Read the model definition and answer for the solid it produces. Units are mm, in the model's axes. Give positions to 0.01 mm unless a question says otherwise; leave off trailing zeros. Answer as a JSON object with one key per item and string values. Group by question number.
```python
from build123d import *

# Parameters (mm, degrees)
SKETCH2_R          = 5.55625
CUT_EXTRUDE1_DEPTH = 141.819693743
CIRPATTERN1_COUNT  = 4
CHAMFER1_SIZE      = 0.508
CHAMFER1_SIZE2     = 3.302
CHAMFER2_SIZE      = 1.5875
FILLET1_R          = 0.762


with BuildPart() as part:
    # Sketch1 → Revolve1 (revolve)
    with BuildSketch(Plane.XY, mode=Mode.PRIVATE) as revolve1_sk:
        Polygon((0, 41.275), (0, 98.425), (21.336, 98.425), (21.336, 70.0151), (25.4, 70.0151), (25.4, 41.275), align=None)
    revolve(revolve1_sk.sketch.rotate(Axis((0, 0, 0), (1, 0, 0)), 90), axis=Axis((0, 0, 0), (1, 0, 0)))

    # Sketch2 → Cut-Extrude1 (cut, through all)
    with BuildSketch(Plane(origin=(21.336, 0, 0), x_dir=(0, 0, -1), z_dir=(1, 0, 0))):
        with Locations((59.494196802, 59.494196802)):
            Circle(SKETCH2_R)
    cut_extrude1 = extrude(amount=-CUT_EXTRUDE1_DEPTH, mode=Mode.SUBTRACT)

    # CirPattern1: Cut-Extrude1 ×4 about axis
    cirpattern1_axis = Axis((0, 0, 0), (1, 0, 0))
    for i in range(1, CIRPATTERN1_COUNT):
        add(cut_extrude1.rotate(cirpattern1_axis, i * 360 / CIRPATTERN1_COUNT), mode=Mode.SUBTRACT)

    # Chamfer1
    chamfer1_edges = [part.edges().sort_by_distance(p)[0] for p in [
        (25.4, 0, -70.0151),
    ]]
    chamfer1_side = [part.faces().sort_by_distance(p)[0] for p in [
        (25.4, 0, -68.03477392),
    ]]
    chamfer(chamfer1_edges, length=CHAMFER1_SIZE, length2=CHAMFER1_SIZE2, reference=chamfer1_side[0])

    # Chamfer2
    chamfer2_edges = [part.edges().sort_by_distance(p)[0] for p in [
        (25.4, 0, -41.275),
    ]]
    chamfer(chamfer2_edges, length=CHAMFER2_SIZE)

    # Fillet1
    fillet1_edges = [part.edges().sort_by_distance(p)[0] for p in [
        (21.336, 0, -70.0151),
    ]]
    fillet(fillet1_edges, radius=FILLET1_R - 0.0001)  # a hair under: the kernel refuses the full size


solid = part.part
```
1) For a pull along Y with two mould halves and no side action, classify faces 1 (the cylindrical face through (10.82, 63.25, -55.4)), 2 (the conical face through (25.19, -58.64, 37.38)), 3 (the flat face through (21.336, -23.3, -67)) as released by +Y, released by -Y, zero draft, split by the parting line, or undercut.
2) Flat-ended cylindrical pins translate along their axes: pin 1 Ø3 at (x, y) = (15.5, -56) entering from +Z; pin 2 Ø6.5 at (y, z) = (59.49, -59.49) entering from -X; pin 3 Ø3 at (x, y) = (21, 56.5) entering from -Z; pin 4 Ø3 at (x, y) = (20, -12.5) entering from -Z. Find the tip coordinate at first contact, or state that the pin passes through.
3) Find the intervals of material crossed by line 1 (Z direction, x = 4.5, y = -2); line 2 (Y direction, x = 14.5, z = 63); line 3 (Y direction, x = 16.25, z = 0) (3 decimals), in increasing order. Write a range as [from, to].
4) Find section C-C, the plane x = 11.75. Give the number of separate pieces and of enclosed holes in the cut face, and give its area (3 significant figures).
Values follow:
{
 "1": {"face 1": "undercut", "face 2": "split by the parting line", "face 3": "zero draft"},
 "2": {"pin 1": "stops at z = 81.96", "pin 2": "passes through", "pin 3": "stops at z = -81.62", "pin 4": "stops at z = -97.81"},
 "3": {"line 1": "z = [-98.4, -41.23], [41.23, 98.4]", "line 2": "y = [-75.62, -63.8], [-55.18, 55.18], [63.8, 75.62]", "line 3": "y = [-98.425, -41.275], [41.275, 98.425]"},
 "4": {"separate pieces": "1", "enclosed holes": "5", "area": "24,700 mm2"}
}
